Could you check a few things on this model? Use its own coordinates, in mm. Round coordinates to 2 decimals unless told otherwise and drop trailing zeros. Return JSON: item names as keys, results as strings. Group by question number.
from build123d import *

# Parameters (mm, degrees)
SKETCH1_R      = 2.6035
SKETCH1_R_2    = 3.3274
EXTRUDE1_DEPTH = 908.05


with BuildPart() as part:
    # Sketch1 → Extrude1 (new body)
    with BuildSketch(Plane.XY):
        with BuildLine():
            Line((23.114, 17.475199816), (23.114, 16.560799816))
            ThreePointArc((23.114, 16.560799816), (23.575248241, 15.447248057), (24.6888, 14.985999816))
            Line((24.6888, 14.985999816), (28.448, 14.985999816))
            ThreePointArc((28.448, 14.985999816), (29.076617928, 14.725617744), (29.337, 14.096999816))
            Line((29.337, 14.096999816), (29.337, 13.528917816))
            ThreePointArc((29.337, 13.528917816), (29.269328904, 13.188712244), (29.076617928, 12.900299887))
            Line((29.076617928, 12.900299887), (24.305516832, 8.129198791))
            ThreePointArc((24.305516832, 8.129198791), (22.76457081, 7.099571576), (20.946901043, 6.73801458))
            Line((20.946901043, 6.73801458), (17.153098957, 6.73801458))
            ThreePointArc((17.153098957, 6.73801458), (15.33542919, 7.099571576), (13.794483168, 8.129198791))
            Line((13.794483168, 8.129198791), (9.023382072, 12.900299887))
            ThreePointArc((9.023382072, 12.900299887), (8.830671096, 13.188712244), (8.763, 13.528917816))
            Line((8.763, 13.528917816), (8.763, 14.096999816))
            ThreePointArc((8.763, 14.096999816), (9.023382072, 14.725617744), (9.652, 14.985999816))
            Line((9.652, 14.985999816), (13.4112, 14.985999816))
            ThreePointArc((13.4112, 14.985999816), (14.524751759, 15.447248057), (14.986, 16.560799816))
            Line((14.986, 16.560799816), (14.986, 17.475199816))
            ThreePointArc((14.986, 17.475199816), (14.524751759, 18.588751575), (13.4112, 19.049999816))
            Line((13.4112, 19.049999816), (-13.4112, 19.049999816))
            ThreePointArc((-13.4112, 19.049999816), (-14.524751759, 18.588751575), (-14.986, 17.475199816))
            Line((-14.986, 17.475199816), (-14.986, 16.560799816))
            ThreePointArc((-14.986, 16.560799816), (-14.524751759, 15.447248057), (-13.4112, 14.985999816))
            Line((-13.4112, 14.985999816), (-9.652, 14.985999816))
            ThreePointArc((-9.652, 14.985999816), (-9.023382072, 14.725617744), (-8.763, 14.096999816))
            Line((-8.763, 14.096999816), (-8.763, 13.528917816))
            ThreePointArc((-8.763, 13.528917816), (-8.830671096, 13.188712244), (-9.023382072, 12.900299887))
            Line((-9.023382072, 12.900299887), (-13.794483168, 8.129198791))
            ThreePointArc((-13.794483168, 8.129198791), (-15.33542919, 7.099571576), (-17.153098957, 6.73801458))
            Line((-17.153098957, 6.73801458), (-20.946901043, 6.73801458))
            ThreePointArc((-20.946901043, 6.73801458), (-22.76457081, 7.099571576), (-24.305516832, 8.129198791))
            Line((-24.305516832, 8.129198791), (-29.076617928, 12.900299887))
            ThreePointArc((-29.076617928, 12.900299887), (-29.269328904, 13.188712244), (-29.337, 13.528917816))
            Line((-29.337, 13.528917816), (-29.337, 14.096999816))
            ThreePointArc((-29.337, 14.096999816), (-29.076617928, 14.725617744), (-28.448, 14.985999816))
            Line((-28.448, 14.985999816), (-24.6888, 14.985999816))
            ThreePointArc((-24.6888, 14.985999816), (-23.575248241, 15.447248057), (-23.114, 16.560799816))
            Line((-23.114, 16.560799816), (-23.114, 17.475199816))
            ThreePointArc((-23.114, 17.475199816), (-23.575248241, 18.588751575), (-24.6888, 19.049999816))
            Line((-24.6888, 19.049999816), (-34.925, 19.049999816))
            ThreePointArc((-34.925, 19.049999816), (-37.17006403, 18.120063846), (-38.1, 15.874999816))
            Line((-38.1, 15.874999816), (-38.1, 3.175))
            ThreePointArc((-38.1, 3.175), (-37.17006403, 0.92993597), (-34.925, 0))
            Line((-34.925, 0), (34.925, 0))
            ThreePointArc((34.925, 0), (37.17006403, 0.92993597), (38.1, 3.175))
            Line((38.1, 3.175), (38.1, 15.874999816))
            ThreePointArc((38.1, 15.874999816), (37.17006403, 18.120063846), (34.925, 19.049999816))
            Line((34.925, 19.049999816), (24.6888, 19.049999816))
            ThreePointArc((24.6888, 19.049999816), (23.575248241, 18.588751575), (23.114, 17.475199816))
        make_face()
        with Locations((-33.909, 14.8082)):
            Circle(SKETCH1_R, mode=Mode.SUBTRACT)
        with Locations((31.75, 6.35)):
            Circle(SKETCH1_R_2, mode=Mode.SUBTRACT)
        with Locations((33.909, 14.8082)):
            Circle(SKETCH1_R, mode=Mode.SUBTRACT)
        with Locations((-31.75, 6.35)):
            Circle(SKETCH1_R_2, mode=Mode.SUBTRACT)
        with BuildLine():
            Line((-9.944292429, 6.232025428), (-6.090184211, 10.086133646))
            ThreePointArc((-6.090184211, 10.086133646), (-5.060556996, 11.627079669), (-4.699, 13.444749436))
            Line((-4.699, 13.444749436), (-4.699, 13.715999816))
            ThreePointArc((-4.699, 13.715999816), (-4.327025612, 14.614025428), (-3.429, 14.985999816))
            Line((-3.429, 14.985999816), (3.429, 14.985999816))
            ThreePointArc((3.429, 14.985999816), (4.327025612, 14.614025428), (4.699, 13.715999816))
            Line((4.699, 13.715999816), (4.699, 13.444749436))
            ThreePointArc((4.699, 13.444749436), (5.060556996, 11.627079669), (6.090184211, 10.086133646))
            Line((6.090184211, 10.086133646), (9.944292429, 6.232025428))
            ThreePointArc((9.944292429, 6.232025428), (10.219593823, 4.847991857), (9.046266817, 4.063999816))
            Line((9.046266817, 4.063999816), (-9.046266817, 4.063999816))
            ThreePointArc((-9.046266817, 4.063999816), (-10.219593823, 4.847991857), (-9.944292429, 6.232025428))
        make_face(mode=Mode.SUBTRACT)
    extrude(amount=-EXTRUDE1_DEPTH)


solid = part.part
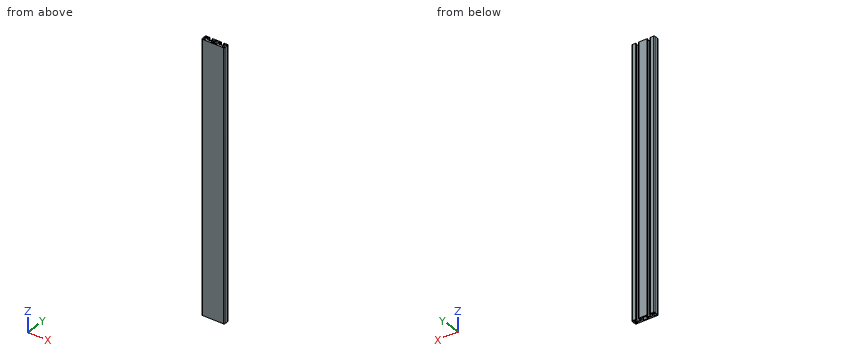
1) Will these pins go through, and if not, where does the flat tip stop? pin 1 (1 mm diameter, centred on y = 17, z = -532, fed in from -X); pin 2 (1.9 mm diameter, centred on x = -18.5, z = -307.5, fed in from +Y); pin 3 (5.5 mm diameter, centred on x = 31.75, y = 6.35, fed in from +Z).
2) I want a section at A-A, the plane z = -473. Give the number of separate pieces and of enclosed holes in the cut face, plus the area to 3 significant figures.
3) If I drill on line 1 along X through (y, z) = (11.5, -672.5); line 2 along Y through (x, z) = (3, -500); line 3 along X through (y, z) = (13.75, -133.5), over which ranges is the centre line in solid material (lowest first)? Write a range as from..to.
Outcome:
{
 "1": {"pin 1": "x = -38.04", "pin 2": "y = 6.74", "pin 3": "through"},
 "2": {"separate pieces": "1", "enclosed holes": "5", "area": "852 mm^2"},
 "3": {"line 1": "-38.1..-27.68, -10.42..-5.12, 5.12..10.42, 27.68..38.1", "line 2": "0..4.06, 14.99..19.05", "line 3": "-38.1..-36.29, -31.53..-29.34, -8.76..-4.7, 4.7..8.76, 29.34..31.53, 36.29..38.1"}
}
